Can you work these out from the model? Positions are in its coordinate system, mm. A direction names the side the tool comes from. Round coordinates to 2 decimals unless told otherwise and drop trailing zeros. Write each loop counter-clockwise with the first axis right and the second up, starting at its lowest first coordinate (ties: lowest second). Pieces come first, ordered by that corner, then holes. Notation, with made-up numbers: M 1.25,-14.75 L 5.25,-14.75 A30 cw 5.25,22.25 Z; hole C -22,-10.75 d2. An arc over 180 degrees is marked long. Answer in a Markdown table with one row per item. Add a question column.
(1) Suppose I cut it at C-C, the plane y = 1.5. Write out the boundary of the cut face in (x, z).
(2) If we mould it in two halves opening along Z, with no side actions, what happens to faces 4 (the face through (22, 5, -5)), 5 (the face through (15, -2, -7)), 6 (the face through (-17, -5, 0.444))? For each: released by +Z, released by -Z, zero draft, split by the parting line, or undercut.
(3) Suppose I cut it at D-D, the plane x = -12. Write out the boundary of the cut face in (y, z).
(4) If I drill on probe 1 along X at (y, z) = (3.5, -6.25); probe 2 along X at (y, z) = (-1.75, -1); probe 3 along Z at (x, y) = (-12, -4.25), over which ranges is the centre line in solid material (lowest first)?
(5) Suppose I cut it at A-A, the plane y = -4.5. Write out the boundary of the cut face in (x, z), then the cut area to 3 significant figures.
(6) Suppose I cut it at B-B, the plane z = 1.75. Write out the boundary of the cut face in (x, y), then the cut area to 3 significant figures.
(7) For faces 1 (the face through (-23.38, 3, -4)), 2 (the face through (21.22, -1.6, -7.2)), 3 (the face through (-17, -6, -1.841)), which set-ups out of +Z, -Z, +X, -X, +Y, -Y let a thin tool reach every point of the face, with its end or its side?
(8) I'm going to push flat-ended pins straight in: pin 1 (5 mm diameter, centred on x = -19, z = -4.5, fed in from -Y); pin 2 (8 mm diameter, centred on x = -10.5, z = -3.5, fed in from +Y); pin 3 (2.5 mm diameter, centred on x = 18, y = -6, fed in from +Z). Where does each tip first touch, or does it pass through?
from build123d import *

# Parameters (mm, degrees)
SKETCH_1_W          = 48
SKETCH_1_H          = 20
EXTRUDE_1_DEPTH     = 5
CUT_EXTRUDE_1_DEPTH = 33.234273685
SKETCH_3_W          = 12
SKETCH_3_H          = 15.07
EXTRUDE_2_DEPTH     = 10
SKETCH_4_W          = 10.5
SKETCH_4_H          = 8
CUT_EXTRUDE_2_DEPTH = 50.294132697


with BuildPart() as part:
    # 草图1 → 凸台-拉伸1 (new body)
    with BuildSketch(Plane(origin=(0, 0, 0), x_dir=(1, 0, 0), z_dir=(0, 1, 0))):
        with Locations((-0.78, 4.625714286)):
            Rectangle(SKETCH_1_W, SKETCH_1_H)
    extrude(amount=EXTRUDE_1_DEPTH)

    # 草图2 → 切除-拉伸1 (cut, through all)
    with BuildSketch(Plane.XY.offset(5.374285714)):
        Polygon((-22.78, 5), (-22.78, 4.5), (-23.38, 4.5), (-23.38, 1), (21.82, 1), (21.82, 4.5), (21.22, 4.5), (21.22, 5), align=None)
    extrude(amount=-CUT_EXTRUDE_1_DEPTH, mode=Mode.SUBTRACT)

    # 草图3 → 凸台-拉伸2 (add)
    with BuildSketch(Plane.XZ):
        with Locations((-16.78, -7.090714286)):
            Rectangle(SKETCH_3_W, SKETCH_3_H)
        with Locations((15.22, -7.090714286)):
            Rectangle(SKETCH_3_W, SKETCH_3_H)
    extrude(amount=EXTRUDE_2_DEPTH)

    # 草图4 → 切除-拉伸2 (cut, through all)
    with BuildSketch(Plane(origin=(21.22, 0, 0), x_dir=(0, 0, -1), z_dir=(1, 0, 0))):
        with Locations((7.090714286, -6)):
            Rectangle(SKETCH_4_W, SKETCH_4_H)
    extrude(amount=-CUT_EXTRUDE_2_DEPTH, mode=Mode.SUBTRACT)


solid = part.part
Calculated:
| question | item | result |
|---|---|---|
| 1 | outline | M -24.78,-14.63 L -23.38,-14.63 L -23.38,5.37 L -24.78,5.37 Z; M 21.82,-14.63 L 23.22,-14.63 L 23.22,5.37 L 21.82,5.37 Z |
| 2 | face 4 | zero draft |
| 2 | face 5 | undercut |
| 2 | face 6 | released by +Z |
| 3 | outline | M -10,-14.63 L 1,-14.63 L 1,5.37 L 0,5.37 L 0,0.44 L -10,0.44 L -10,-1.84 L -2,-1.84 L -2,-12.34 L -10,-12.34 Z |
| 4 | probe 1 | -24.78 to -23.38, 21.82 to 23.22 |
| 4 | probe 2 | -22.78 to -10.78, 9.22 to 21.22 |
| 4 | probe 3 | -14.63 to -12.34, -1.84 to 0.44 |
| 5 | outline | M -22.78,-14.63 L -10.78,-14.63 L -10.78,-12.34 L -22.78,-12.34 Z; M -22.78,-1.84 L -10.78,-1.84 L -10.78,0.44 L -22.78,0.44 Z; M 9.22,-14.63 L 21.22,-14.63 L 21.22,-12.34 L 9.22,-12.34 Z; M 9.22,-1.84 L 21.22,-1.84 L 21.22,0.44 L 9.22,0.44 Z |
| 5 | area | 110 mm² |
| 6 | outline | M -24.78,0 L 23.22,0 L 23.22,5 L 21.22,5 L 21.22,4.5 L 21.82,4.5 L 21.82,1 L -23.38,1 L -23.38,4.5 L -22.78,4.5 L -22.78,5 L -24.78,5 Z |
| 6 | area | 59.8 mm² |
| 7 | face 1 | +Z, -Z |
| 7 | face 2 | +Z, -Z, +X, -Y |
| 7 | face 3 | +X, -X, -Y |
| 8 | pin 1 | y = -2 |
| 8 | pin 2 | y = 1 |
| 8 | pin 3 | z = 0.44 |
